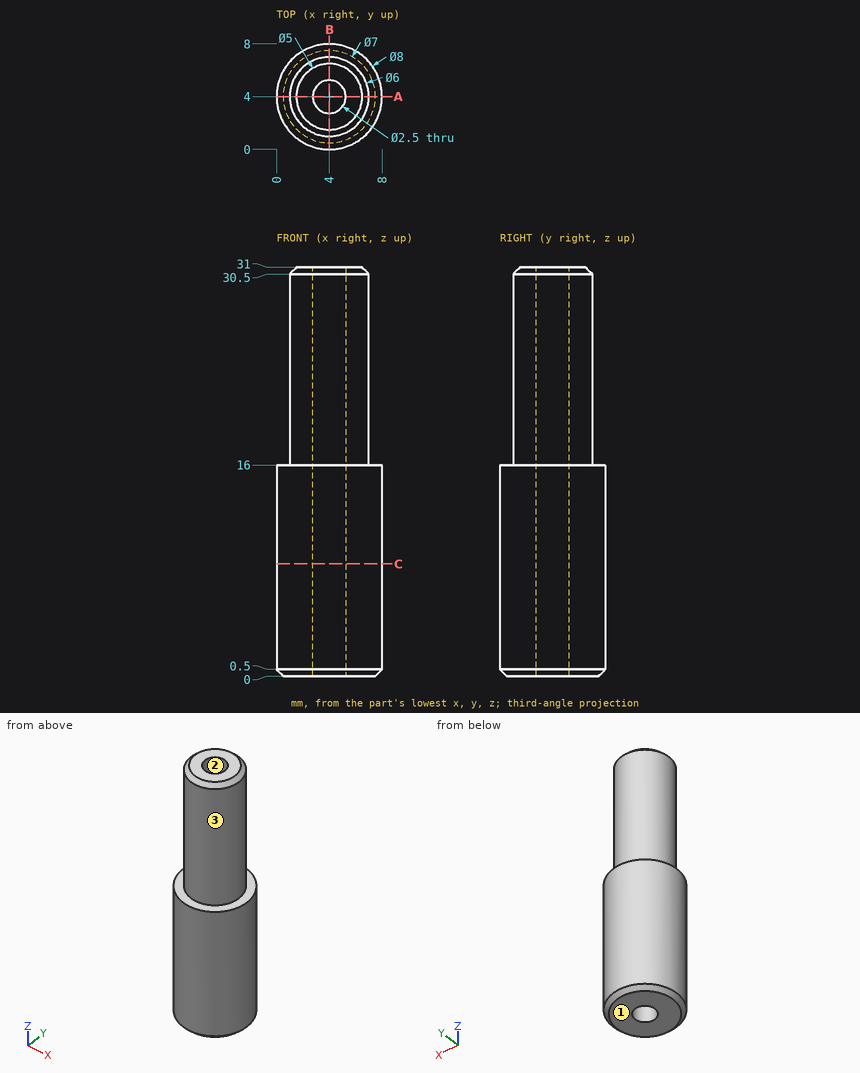
Job drawing, mm, ordinate dimensions from the low corner. One solid piece. Round coordinates to 2 decimals unless told otherwise and drop trailing zeros. Loops run counter-clockwise (first coordinate to the right, second up) from the corner with the lowest first, then second, coordinate; pieces in that order, holes last.
(1) Drop flat-ended pins along their axis: pin 1 (2 mm diameter, centred on x = 4, y = 4, fed in from +Z); pin 2 (4 mm diameter, centred on x = 4.5, z = 18.5, fed in from +Y); pin 3 (1.5 mm diameter, centred on x = 5.5, z = 25, fed in from -Y); pin 4 (3 mm diameter, centred on y = 2.5, z = 21, fed in from +X). Give the stop position or say it passes through.
(2) Cut at C-C (z = 8.5). Give the cut face in (x, y).
(3) Cut at A-A (y = 4). Give the cut face in (x, z), plus the area to 3 significant figures.
(4) Wall check: line 1 along Y through (x, z) = (4, 23); line 2 along Y through (x, z) = (4.5, 6); line 3 along X through (y, z) = (3, 15). Give the ranges that are in metal, low to high.
(5) Two-plate mould, pull along Y, no slides. Class the marked faces 1, 2 and 3: +Y half, -Y half, draft (parallel to the pull), parting line (faces both ways), or undercut.
Findings below:
1. pin 1: passes through
1. pin 2: stops at y = 7
1. pin 3: stops at y = 1.1
1. pin 4: stops at x = 7
2. outline: circle Ø8 at (4, 4); hole circle Ø2.5 at (4, 4)
3. outline: (0, 0.5) - (0.5, 0) - (2.75, 0) - (2.75, 31) - (1.5, 31) - (1, 30.5) - (1, 16) - (0, 16) - close; (5.25, 0) - (7.5, 0) - (8, 0.5) - (8, 16) - (7, 16) - (7, 30.5) - (6.5, 31) - (5.25, 31) - close
3. area: 140 mm2
4. line 1: y = 1 to 2.75, 5.25 to 7
4. line 2: y = 0.03 to 2.85, 5.15 to 7.97
4. line 3: x = 0.13 to 3.25, 4.75 to 7.87
5. face 1: draft
5. face 2: undercut
5. face 3: parting line
